from build123d import *

# Parameters (mm, degrees)
BOSS_EXTRUDE1_DEPTH                            = 1.62814
CSK_FOR_M3_5_FLAT_HEAD_MACHINE_SCREW1_AT_COUNT = 2
CSK_FOR_M3_5_FLAT_HEAD_MACHINE_SCREW1_AT_PITCH = 35.6


with BuildPart() as part:
    # Sketch1 → Boss-Extrude1 (new body)
    with BuildSketch(Plane(origin=(0, 0, 31.399786773), x_dir=(-1, 0, 0), z_dir=(0, 0, -1))):
        with BuildLine():
            Line((16.918894582, 11.465), (-17.711105418, 11.465))
            ThreePointArc((-17.711105418, 11.465), (-20.468821865, 10.322716447), (-21.611105418, 7.565))
            Line((-21.611105418, 7.565), (-21.611105418, -7.565))
            ThreePointArc((-21.611105418, -7.565), (-20.468821865, -10.322716447), (-17.711105418, -11.465))
            Line((-17.711105418, -11.465), (16.918894582, -11.465))
            ThreePointArc((16.918894582, -11.465), (19.676611029, -10.322716447), (20.818894582, -7.565))
            Line((20.818894582, -7.565), (20.818894582, 7.565))
            ThreePointArc((20.818894582, 7.565), (19.676611029, 10.322716447), (16.918894582, 11.465))
        make_face()
    extrude(amount=-BOSS_EXTRUDE1_DEPTH)

    # Sketch2 → CSK for M3.5 Flat Head Machine Screw1 (revolve, cut)
    with BuildSketch(Plane(origin=(-17.403894582, 0, 33.027926773), x_dir=(0, -1, 0), z_dir=(1, 0, 0))):
        Polygon((0, 0), (0, 1.62814), (2.0955, 1.62814), (2.0955, 0.94962912), (2.921, 0), align=None)
    csk_for_m3_5_flat_head_machine_screw1 = revolve(axis=Axis((-17.403894582, 0, 39.377926773), (0, 0, -1)), mode=Mode.SUBTRACT)

    # CSK for M3.5 Flat Head Machine Screw1 at: CSK for M3.5 Flat Head Machine Screw1 ×2
    with Locations(*[(i * CSK_FOR_M3_5_FLAT_HEAD_MACHINE_SCREW1_AT_PITCH, 0, 0) for i in range(1, CSK_FOR_M3_5_FLAT_HEAD_MACHINE_SCREW1_AT_COUNT)]):
        add(csk_for_m3_5_flat_head_machine_screw1, mode=Mode.SUBTRACT)


solid = part.part
Can you work these out from the model? Positions are in its coordinate system, mm. Round coordinates to 2 decimals unless told otherwise and drop trailing zeros. Write each loop counter-clockwise with the first axis right and the second up, starting at its lowest first coordinate (ties: lowest second). Pieces come first, ordered by that corner, then holes. Notation, with made-up numbers: M 15,53.5 L 69,53.5 A22 cw 69,62.5 Z; hole C 55.5,38 d8. An arc over 180 degrees is marked long. Use a Markdown table: item, result.
Item 1: I want a section at C-C (y = -9.25). List the corners of the cut face in (x, z) for me.
Found:
| item | result |
|---|---|
| outline | M -20.44,31.4 L 21.23,31.4 L 21.23,33.03 L -20.44,33.03 Z |
Item 2: I want a section at B-B (z = 31.7). List the corners of the cut face in (x, y) for me (1 decimal), and give its area (3 significant figures).
Found:
| item | result |
|---|---|
| outline | M -20.8,-7.6 A3.9 ccw -16.9,-11.5 L 17.7,-11.5 A3.9 ccw 21.6,-7.6 L 21.6,7.6 A3.9 ccw 17.7,11.5 L -16.9,11.5 A3.9 ccw -20.8,7.6 Z; hole C -17.4,0 d4.2; hole C 18.2,0 d4.2 |
| area | 932 mm2 |
Item 3: I want a section at A-A (y = 0). List the corners of the cut face in (x, z) for me.
Found:
| item | result |
|---|---|
| outline | M -20.82,31.4 L -19.5,31.4 L -19.5,32.08 L -20.32,33.03 L -20.82,33.03 Z; M -15.31,31.4 L 16.1,31.4 L 16.1,32.08 L 15.28,33.03 L -14.48,33.03 L -15.31,32.08 Z; M 20.29,31.4 L 21.61,31.4 L 21.61,33.03 L 21.12,33.03 L 20.29,32.08 Z |
Item 4: For pin 1 Ø5 at (x, y) = (18.2, 0) entering from -Z; pin 2 Ø5 at (x, y) = (-17.4, 0) entering from +Z, each with a flat end and sliding along its axis, tell me the tip position at first contact or that it passes through.
Found:
| item | result |
|---|---|
| pin 1 | stops at z = 31.4 |
| pin 2 | stops at z = 32.55 |
Item 5: We'd pull the mould along Y, two halves only. Please class faces 1 (the face through (1, 0, 33.028)), 2 (the face through (16.12, 0.27, 31.74)), 3 (the face through (-19.6, -10.4, 32.2)), 4 (the face through (-19.48, 0.27, 31.74)): released by +Y, released by -Y, zero draft, split by the parting line, or undercut.
Found:
| item | result |
|---|---|
| face 1 | zero draft |
| face 2 | undercut |
| face 3 | released by -Y |
| face 4 | undercut |
Item 6: If I drill on line 1 along X through (y, z) = (0, 31.6); line 2 along X through (y, z) = (-2, 32.95); line 3 along Y through (x, z) = (18.5, 32.7), over which ranges is the centre line in solid material (lowest first)? Write a range as [from, to].
Found:
| item | result |
|---|---|
| line 1 | x = [-20.82, -19.5], [-15.31, 16.1], [20.29, 21.61] |
| line 2 | x = [-20.82, -19.44], [-15.37, 16.16], [20.23, 21.61] |
| line 3 | y = [-11.38, -2.62], [2.62, 11.38] |
